Could you check a few things on this model? Use its own coordinates, in mm. A direction names the side the tool comes from. Coordinates: 2 decimals unless noted, no trailing zeros. Loops run counter-clockwise (first coordinate to the right, second up) from the corner with the lowest first, then second, coordinate; pieces in that order, holes last.
1) If I drill on line 1 along Z through (x, y) = (68, 13.5); line 2 along Y through (x, z) = (0, 1.4); line 3 along Y through (x, z) = (0, 3), over which ranges is the centre line in solid material (lowest first)?
2) Will these pins go through, and if not, where does the flat tip stop? P1, Ø12, axis at x = -28.28, y = 28.28, coming from the -Z side; P2, Ø4, axis at x = -2.5, y = -0.5, coming from the -Z side; P3, Ø3, axis at x = 34, z = -80, coming from the +Y side; P4, Ø1.5, axis at y = -47, z = -95, coming from the -X side.
3) Thinking about a two-plate mould opening in X: for faces 1 (the face through (48, -27, -120)), 2 (the face through (-2.17, -49.76, 2.46)), 3 (the face through (-55.65, 26.24, -59.16)), which applies, released by +X, released by -X, zero draft, split by the parting line, or undercut?
4) Imagine slicing it at C-C on z = -106. Please give me the cut outline in (x, y).
5) For faces 4 (the face through (-48, 26, -120)), 5 (the face through (47.18, -34, -59.16)), which set-ups out of +Z, -Z, +X, -X, +Y, -Y let a thin tool reach every point of the face, with its end or its side?
6) Imagine slicing it at A-A on x = 0. Give the number of separate pieces and of enclosed holes in the cut face, plus the area to 3 significant figures.
```python
from build123d import *

# Parameters (mm, degrees)
F0_R     = 75
F0_R_2   = 10
F1_DEPTH = 5
F2_R     = 4.99999
F3_R     = 7.5
F4_DEPTH = 120


# Not quite as in the source:
# - a fillet or chamfer is up to 0.001 mm smaller than in the source, because OpenCascade refuses the exact size


with BuildPart() as f1:
    # F0 (on Top) → F1 (new body)
    with BuildSketch(Plane.XY):
        Circle(F0_R)
        with Locations((-28.2842712475, -28.2842712475)):
            Circle(F0_R_2, mode=Mode.SUBTRACT)
        with Locations((0, -40)):
            Circle(F0_R_2, mode=Mode.SUBTRACT)
        with Locations((28.2842712475, -28.2842712475)):
            Circle(F0_R_2, mode=Mode.SUBTRACT)
        with Locations((-40, 0)):
            Circle(F0_R_2, mode=Mode.SUBTRACT)
        with Locations((-28.2842712475, 28.2842712475)):
            Circle(F0_R_2, mode=Mode.SUBTRACT)
        with Locations((28.2842712475, 28.2842712475)):
            Circle(F0_R_2, mode=Mode.SUBTRACT)
        with Locations((40, 0)):
            Circle(F0_R_2, mode=Mode.SUBTRACT)
        with Locations((0, 40)):
            Circle(F0_R_2, mode=Mode.SUBTRACT)
    extrude(amount=F1_DEPTH)

    # F2 (radius 5 in the source; OpenCascade refuses exactly that, so slightly less here)
    f2_edges = [f1.edges().sort_by_distance(p)[0] for p in [
        (-75, 0, 5),
    ]]
    fillet(f2_edges, radius=F2_R)

    # F3 (on face) → F4 (join)
    with BuildSketch(Plane(origin=(0, 0, 0), x_dir=(1, 0, 0), z_dir=(0, 0, -1))):
        with Locations((-26.565498142, 48.1588445508)):
            Circle(F3_R)
        with Locations((-48.1588445508, -26.565498142)):
            Circle(F3_R)
        with Locations((26.565498142, -48.1588445508)):
            Circle(F3_R)
        with Locations((48.1588445508, 26.565498142)):
            Circle(F3_R)
    extrude(amount=F4_DEPTH)


solid = f1.part
```
Filled in:
1. line 1: z = 0 to 5
1. line 2: y = -74.8 to -50, -30 to 30, 50 to 74.8
1. line 3: y = -74 to -50, -30 to 30, 50 to 74
2. P1: passes through
2. P2: stops at z = 0
2. P3: stops at y = 52.74
2. P4: stops at x = -34.05
3. face 1: zero draft
3. face 2: undercut
3. face 3: split by the parting line
4. outline: circle Ø15 at (-48.16, 26.57); circle Ø15 at (-26.57, -48.16); circle Ø15 at (26.57, 48.16); circle Ø15 at (48.16, -26.57)
5. face 4: -Z, +X, -X, +Y, -Y
5. face 5: -Z
6. separate pieces: 3
6. enclosed holes: 0
6. area: 539 mm2
